Design review of the part built by this model. Coordinates are the model's own, in mm. A direction names the side the tool comes from. Coordinates: 2 decimals unless noted, no trailing zeros. Loops run counter-clockwise (first coordinate to the right, second up) from the corner with the lowest first, then second, coordinate; pieces in that order, holes last. Notation, with made-up numbers: (23, -6.5) - (44, -6.5) arc R25 cw to (44, 23.5) - close; hole circle Ø5 at (10, 40). An arc over 180 degrees is marked (long way). One line per question, with ' | ' between items.
from build123d import *

# Parameters (mm, degrees)
BOSS_EXTRUDE3_DEPTH     = 38.1
SHELL1_T                = -1.27
CUT_EXTRUDE1_DEPTH      = 39.1
SKETCH4_R               = 2
CUT_EXTRUDE2_DEPTH      = 2.54
SKETCH5_W               = 15
SKETCH5_H               = 28.1
CUT_EXTRUDE3_DEPTH      = 18.025
CUT_EXTRUDE3_DEPTH_BACK = 21
SKETCH6_W               = 7.5
SKETCH6_H               = 38.1
BOSS_EXTRUDE4_DEPTH     = 2.54


with BuildPart() as part:
    # Sketch1 → Boss-Extrude3 (new body)
    with BuildSketch(Plane.XY):
        with BuildLine():
            Line((-22.5, 0), (-22.5, -20))
            Line((-22.5, -20), (22.5, -20))
            Line((22.5, -20), (22.5, 0))
            ThreePointArc((22.5, 0), (0, 17.025), (-22.5, 0))
        make_face()
    extrude(amount=BOSS_EXTRUDE3_DEPTH)

    # Shell1
    shell1_openings = [part.faces().sort_by_distance(p)[0] for p in [
        (0, -20, 19.05),
    ]]
    offset(amount=SHELL1_T, openings=shell1_openings, kind=Kind.INTERSECTION)

    # Sketch3 → Cut-Extrude1 (cut, through all)
    with BuildSketch(Plane(origin=(0, 0, 0), x_dir=(-1, 0, 0), z_dir=(0, 0, -1))):
        with BuildLine():
            Line((-4.5, 10), (-4.5, -20))
            Line((-4.5, -20), (4.5, -20))
            Line((4.5, -20), (4.5, 10))
            ThreePointArc((4.5, 10), (0, 14.5), (-4.5, 10))
        make_face()
    extrude(amount=-CUT_EXTRUDE1_DEPTH, mode=Mode.SUBTRACT)

    # Sketch4 → Cut-Extrude2 (cut)
    with BuildSketch(Plane(origin=(0, 0, 0), x_dir=(-1, 0, 0), z_dir=(0, 0, -1))):
        with Locations((-17.5, 0)):
            Circle(SKETCH4_R)
        with Locations((17.5, 0)):
            Circle(SKETCH4_R)
    extrude(amount=-CUT_EXTRUDE2_DEPTH, mode=Mode.SUBTRACT)

    # Sketch5 → Cut-Extrude3 (cut, two sides)
    with BuildSketch(Plane(origin=(0, 0, 0), x_dir=(1, 0, 0), z_dir=(0, 1, 0))) as cut_extrude3_sk:
        with Locations((0, -19.05)):
            Rectangle(SKETCH5_W, SKETCH5_H)
    extrude(amount=CUT_EXTRUDE3_DEPTH, mode=Mode.SUBTRACT)
    extrude(cut_extrude3_sk.sketch, amount=-CUT_EXTRUDE3_DEPTH_BACK, mode=Mode.SUBTRACT)

    # Sketch6 → Boss-Extrude4 (add)
    with BuildSketch(Plane.XZ.offset(20)):
        with Locations((-26.25, 19.05)):
            Rectangle(SKETCH6_W, SKETCH6_H)
        with Locations((26.25, 19.05)):
            Rectangle(SKETCH6_W, SKETCH6_H)
    extrude(amount=-BOSS_EXTRUDE4_DEPTH)


solid = part.part
Q1. Draft analysis for pull direction Z (two halves, no side actions). For faces 1 (the flat face through (6, -6, 38.1)), 2 (the flat face through (-5, -6, 36.83)), 3 (the flat face through (-22.5, -9, 19)), state which applies: +Z half, -Z half, draft (parallel to the pull), parting line (faces both ways), or undercut.
Returned:
face 1: +Z half | face 2: undercut | face 3: draft
Q2. To check wall thickness, follow line 1 along Z through (x, y) = (9.5, 8.5); line 2 along X through (y, z) = (-12.5, 24); line 3 along Y through (x, z) = (17.5, 0.3). State the ranges of each line that lie inside material, in increasing order.
Returned:
line 1: z = 0 to 1.27, 36.83 to 38.1 | line 2: x = -22.5 to -21.23, 21.23 to 22.5 | line 3: y = -20 to -2, 2 to 9.15
Q3. Tool access review of faces 4 (the flat face through (-21.23, -10, 19)), 5 (the cylindrical face through (-15.9, -1.2, 0.6)), 6 (the flat face through (-4.5, -5, 1)), 7 (the flat face through (-26, -17.46, 19)): name each direction out of +Z, -Z, +X, -X, +Y, -Y from which nothing blocks a thin tool from reaching the whole face with its end or side.
Returned:
face 4: -Y | face 5: -Z | face 6: +Z, -Z, -Y | face 7: +Z, -Z, -X, +Y
Q4. Take a section at C-C (x = 0). Give the boundary of the cut face in (y, z) (3 decimals).
Returned:
outline: (14.5, 0) - (17.025, 0) - (17.025, 5) - (15.755, 5) - (15.755, 1.27) - (14.5, 1.27) - close; (14.5, 36.83) - (15.755, 36.83) - (15.755, 33.1) - (17.025, 33.1) - (17.025, 38.1) - (14.5, 38.1) - close
Q5. Take a section at B-B (y = -10). Give the boundary of the cut face in (x, z), plus the area to 3 significant figures.
Returned:
outline: (-22.5, 0) - (-4.5, 0) - (-4.5, 1.27) - (-21.23, 1.27) - (-21.23, 36.83) - (-4.5, 36.83) - (-4.5, 38.1) - (-22.5, 38.1) - close; (4.5, 0) - (22.5, 0) - (22.5, 38.1) - (4.5, 38.1) - (4.5, 36.83) - (21.23, 36.83) - (21.23, 1.27) - (4.5, 1.27) - close | area: 182 mm²
Q6. For pin 1 (12 mm diameter, centred on x = 15.5, z = 31, fed in from +Y); pin 2 (10 mm diameter, centred on y = -12, z = 19.5, fed in from +X); pin 3 (2 mm diameter, centred on x = -27, z = 10.5, fed in from +Y), all flat-tipped, find the tip position at first contact; note any pin that passes through.
Returned:
pin 1: stops at y = 15.01 | pin 2: stops at x = 22.5 | pin 3: stops at y = -17.46
Q7. Take a section at A-A (z = 7). Give the boundary of the cut face in (x, y).
Returned:
outline: (-30, -20) - (-21.23, -20) - (-21.23, -0.18) arc R22.11 cw to (-7.5, 14.44) - (-7.5, 15.79) arc R23.38 ccw to (-22.5, 0) - (-22.5, -17.46) - (-30, -17.46) - close; (7.5, 14.44) arc R22.11 cw to (21.23, -0.18) - (21.23, -20) - (30, -20) - (30, -17.46) - (22.5, -17.46) - (22.5, 0) arc R23.38 ccw to (7.5, 15.79) - close
Q8. Take a section at D-D (z = 34). Give the boundary of the cut face in (x, y), plus the area to 3 significant figures.
Returned:
outline: (-30, -20) - (-21.23, -20) - (-21.23, -0.18) arc R22.11 cw to (21.23, -0.18) - (21.23, -20) - (30, -20) - (30, -17.46) - (22.5, -17.46) - (22.5, 0) arc R23.38 ccw to (-22.5, 0) - (-22.5, -17.46) - (-30, -17.46) - close | area: 163 mm²
